Part model, mm, in its own coordinate system. A direction names the side the tool comes from. Round coordinates to 2 decimals unless told otherwise and drop trailing zeros. Order: outer loops, then holes, each group sorted by start corner. A loop starts at its lowest first (then second) coordinate and runs counter-clockwise, first axis right, second up. Notation, with made-up numbers: (21.5, 30) - (56.5, 30) arc R30 ccw to (56.5, 67) - close; hole circle Ø6 at (70, 42). An arc over 180 degrees is marked (long way). Answer as a JSON object with one key per item and string values.
```python
from build123d import *

# Parameters (mm, degrees)
F1_DEPTH = 25.4


with BuildPart() as f1:
    # F0 (on Front) → F1 (new body)
    with BuildSketch(Plane.XZ):
        Polygon((-41.2195250034, 60.3447593749), (-63.4445250034, 60.3447593749), (-64.4639437478, 58.6040624199), (-96.9131098717, 3.1958555594), (-64.3884492879, -53.953048256), (-41.960131377, -53.953048256), (-41.960131377, -41.253048256), (-9.4695250034, -41.253048256), (-9.4695250034, -53.953048256), (15.9304749966, -53.953048256), (15.9304749966, -41.253048256), (47.6804749966, -41.253048256), (47.6804749966, -53.953048256), (60.11830526, -53.953048256), (93.5868901283, 3.1958555594), (61.0622295445, 60.3447593749), (47.6804749966, 60.3447593749), (47.6804749966, 47.6447593749), (15.9304749966, 47.6447593749), (15.9304749966, 60.3447593749), (-9.4695250034, 60.3447593749), (-9.4695250034, 47.6447593749), (-41.2195250034, 47.6447593749), align=None)
        Polygon((-53.7397041917, 23.8567902654), (-9.4695250034, 23.8567902654), (-9.4695250034, -14.2432097346), (-63.4445250034, -14.2432097346), (-63.4445250034, 23.8567902654), align=None, mode=Mode.SUBTRACT)
        Polygon((18.3994676918, -15.853048256), (18.3994676918, 22.246951744), (56.8952597678, 22.246951744), (72.3744676918, 22.246951744), (72.3744676918, -15.853048256), align=None, mode=Mode.SUBTRACT)
    extrude(amount=F1_DEPTH)


solid = f1.part
```
Item 1: Cut at D-D (x = 22). Write the cut outline in (y, z), plus the area to 3 significant figures.
Taken from the geometry:
{"outline": "(-25.4, -41.25) - (0, -41.25) - (0, -15.85) - (-25.4, -15.85) - close; (-25.4, 22.25) - (0, 22.25) - (0, 47.64) - (-25.4, 47.64) - close", "area": "1,290 mm2"}
Item 2: Tool access for faces 1 (the flat face through (76.618, -12.522, -25.779)), 2 (the flat face through (-9.47, -13, -48)), 3 (the flat face through (47.68, -13, 54)), 4 (the flat face through (-9.47, -13, 5)), 5 (the flat face through (54, -13, -53.953)): list every direction of +Z, -Z, +X, -X, +Y, -Y with a clear straight run to the whole face (end or side of a thin tool).
Taken from the geometry:
{"face 1": "-Z, +X, +Y, -Y", "face 2": "-Z, +Y, -Y", "face 3": "+Z, +Y, -Y", "face 4": "+Y, -Y", "face 5": "-Z, +X, -X, +Y, -Y"}
Item 3: Cut at A-A (x = -54.5). Write the cut outline in (y, z).
Taken from the geometry:
{"outline": "(-25.4, -53.95) - (0, -53.95) - (0, -14.24) - (-25.4, -14.24) - close; (-25.4, 23.86) - (0, 23.86) - (0, 60.34) - (-25.4, 60.34) - close"}
Item 4: Two-plate mould, pull along Z, no slides. Class faces 6 (the flat face through (3, -13, -53.953)), 7 (the flat face through (32, -13, 47.645)), 8 (the flat face through (18.399, -13, 3)): pulls with the +Z half, pulls with the -Z half, needs draft (parallel to the pull), parting line crosses it, or undercut.
Taken from the geometry:
{"face 6": "pulls with the -Z half", "face 7": "pulls with the +Z half", "face 8": "undercut"}
Item 5: Drop flat-ended pins along their axis: P1, Ø4, axis at y = -17, z = 56, coming from the -X side; P2, Ø10, axis at y = -8.5, z = 51.5, coming from the +X side; P3, Ø4, axis at y = -12, z = -45, coming from the -X side; P4, Ø1, axis at x = 2, z = 17, coming from the +Y side. Give the stop position or say it passes through.
Taken from the geometry:
{"P1": "x = -67.16", "P2": "x = 68.94", "P3": "x = -70.62", "P4": "y = 0"}
Item 6: Cut at B-B (y = -8.75). State how many separate pieces and enclosed holes the cut face has, plus the area to 3 significant figures.
Taken from the geometry:
{"separate pieces": "1", "enclosed holes": "2", "area": "12,300 mm2"}
Item 7: Cut at C-C (z = 1). Write the cut outline in (x, y), plus the area to 3 significant figures.
Taken from the geometry:
{"outline": "(-95.66, -25.4) - (-63.44, -25.4) - (-63.44, 0) - (-95.66, 0) - close; (-9.47, -25.4) - (18.4, -25.4) - (18.4, 0) - (-9.47, 0) - close; (72.37, -25.4) - (92.3, -25.4) - (92.3, 0) - (72.37, 0) - close", "area": "2,030 mm2"}
Item 8: Probe L1, parallel to Z at x = -60, y = -3; L2, parallel to Z at x = -19, y = -19.75; L3, parallel to X at y = -2, z = 53. List the from-to ranges inside material, lowest first. Write a range as from..to.
Taken from the geometry:
{"L1": "-53.95..-14.24, 23.86..60.34", "L2": "-41.25..-14.24, 23.86..47.64", "L3": "-67.75..-41.22, -9.47..15.93, 47.68..65.24"}
